Verification items for the finished model (mm, model axes). A direction names the side the tool comes from. Coordinates: 2 decimals unless noted, no trailing zeros. Order: outer loops, then holes, each group sorted by start corner. A loop starts at its lowest first (then second) coordinate and runs counter-clockwise, first axis right, second up. Notation, with made-up numbers: (9, 15.25) -> (45, 15.25) arc R25 ccw to (45, 29.25) -> close; hole circle Ø3 at (64.5, 34). An arc over 180 degrees is marked (long way). Use CSV: the item, a comma, the result in double quotes. Start each with the question number.
1) Scan lines: line 1 along X through (y, z) = (-4.5, 1.5); line 2 along Y through (x, z) = (10, 0.5); line 3 along X through (y, z) = (18, 1.75). Record each from-to range of solid material in increasing order.
2) Sectioned sample at A-A on x = 10. Record the boundary of the cut face in (y, z).
3) Go/stop test with flat-tipped pins: pin 1 (2.5 mm diameter, centred on x = -18.43, y = 21.91, fed in from +Z); pin 2 (1.8 mm diameter, centred on x = -18.43, y = -4.09, fed in from +Z); pin 3 (0.8 mm diameter, centred on x = -7.5, z = 0.5, fed in from -Y). Record where each tip stops, or that it passes through.
4) Tool access check on faces 1 (the flat face through (-1.103, -0.079, 0.986)), 2 (the cylindrical face through (14.774, -7.935, 1.699)), 3 (the cylindrical face through (17.6, -8.808, 1.699)). Record the directions out of +Z, -Z, +X, -X, +Y, -Y that give a thin tool (end or side, any length) a straight path to the whole face; none if there is none.
5) Sectioned sample at B-B on z = 1.7. Give the number of separate pieces and of enclosed holes in the cut face, then the cut area to 3 significant figures.
6) Release check for a two-part mould opening along X. For faces 4 (the cylindrical face through (-19.456, -8.808, 1.699)), 5 (the flat face through (-16.6, -8.3, 0.5)), 6 (the cylindrical face through (10.59, -3.31, 0.99)), 7 (the flat face through (19.572, 8.1, 0.5)) record: released by +X, released by -X, zero draft, split by the parting line, or undercut.
7) Sectioned sample at C-C on y = 0. Record the boundary of the cut face in (x, z), then the cut area to 3 significant figures.
from build123d import *

# Parameters (mm, degrees)
SKETCH_1_R          = 1.1
SKETCH_1_W          = 21
SKETCH_1_H          = 14
EXTRUDE_1_DEPTH     = 2
FILLET_2_R          = 1
SKETCH_11_R         = 1
CUT_EXTRUDE_1_DEPTH = 33.917032345
CHAMFER_1_SIZE      = 2


with BuildPart() as part:
    # 草图1 → 凸台-拉伸1 (new body)
    with BuildSketch(Plane.XY):
        Polygon((-21.428351104, 24.906962627), (19.571648896, 24.906962627), (19.571648896, -9.093037373), (17.69677195, -9.093037373), (15.571648896, -9.093037373), (13.89965532, -7.493037373), (-15.756357529, -7.493037373), (-17.428351104, -9.093037373), (-21.428351104, -9.093037373), align=None)
        with Locations((-11.428351104, 18.906962627)):
            Circle(SKETCH_1_R, mode=Mode.SUBTRACT)
        with Locations((-11.428351104, -2.893037373)):
            Circle(SKETCH_1_R, mode=Mode.SUBTRACT)
        with Locations((9.571648896, 18.906962627)):
            Circle(SKETCH_1_R, mode=Mode.SUBTRACT)
        with Locations((9.571648896, -2.893037373)):
            Circle(SKETCH_1_R, mode=Mode.SUBTRACT)
        with Locations((-0.928351104, 7.906962627)):
            Rectangle(SKETCH_1_W, SKETCH_1_H, mode=Mode.SUBTRACT)
    extrude(amount=EXTRUDE_1_DEPTH)

    # 圆角2
    fillet_2_edges = [part.edges().sort_by_distance(p)[0] for p in [
        (-16.592354317, -8.293037373, 2),
        (-0.928351104, -7.493037373, 2),
        (14.735652108, -8.293037373, 2),
        (17.571648896, -9.093037373, 2),
        (19.571648896, 7.906962627, 2),
        (-0.928351104, 24.906962627, 2),
        (-21.428351104, 7.906962627, 2),
        (-19.428351104, -9.093037373, 2),
    ]]
    fillet(fillet_2_edges, radius=FILLET_2_R)

    # 草图11 → 切除-拉伸1 (cut, through all)
    with BuildSketch(Plane.XY.offset(2)):
        with Locations((-18.428351104, 21.906962627)):
            Circle(SKETCH_11_R)
        with Locations((-18.428351104, -4.093037373)):
            Circle(SKETCH_11_R)
        with Locations((16.571648896, 21.906962627)):
            Circle(SKETCH_11_R)
        with Locations((16.571648896, -4.093037373)):
            Circle(SKETCH_11_R)
    extrude(amount=-CUT_EXTRUDE_1_DEPTH, mode=Mode.SUBTRACT)

    # 倒角1
    chamfer_1_edges = [part.edges().sort_by_distance(p)[0] for p in [
        (-0.928351104, 0.906962627, 2),
        (9.571648896, 7.906962627, 2),
        (-11.428351104, 7.906962627, 2),
        (-0.928351104, 14.906962627, 2),
    ]]
    chamfer(chamfer_1_edges, length=CHAMFER_1_SIZE - 0.0001)  # a hair under: the kernel refuses the full size


solid = part.part
Answers follow:
1,line 1,"x = -21.29 to -19.34, -17.51 to 15.66, 17.49 to 19.44"
1,line 2,"y = -7.49 to -3.91, -1.88 to 0.41, 15.41 to 17.89, 19.92 to 24.91"
1,line 3,"x = -21.09 to -12.05, -10.81 to 8.95, 10.19 to 19.23"
2,outline,"(-7.49, 0) -> (-3.91, 0) -> (-3.91, 2) -> (-6.49, 2) arc R1 ccw to (-7.49, 1) -> close; (-1.88, 0) -> (17.89, 0) -> (17.89, 2) -> (16.91, 2) -> (15.34, 0.43) -> (0.48, 0.43) -> (-1.09, 2) -> (-1.88, 2) -> close; (19.92, 0) -> (24.91, 0) -> (24.91, 1) arc R1 ccw to (23.91, 2) -> (19.92, 2) -> close"
3,pin 1,"stops at z = 2"
3,pin 2,"passes through"
3,pin 3,"stops at y = -7.49"
4,face 1,"+Z"
4,face 2,"+Z, -Y"
4,face 3,"+Z, +X, -X, -Y"
5,separate pieces,"1"
5,enclosed holes,"9"
5,area,"849 mm²"
6,face 4,"zero draft"
6,face 5,"undercut"
6,face 6,"undercut"
6,face 7,"released by +X"
7,outline,"(-21.43, 0) -> (19.57, 0) -> (19.57, 1) arc R1 ccw to (18.57, 2) -> (11.57, 2) -> (10.48, 0.91) -> (-12.34, 0.91) -> (-13.43, 2) -> (-20.43, 2) arc R1 ccw to (-21.43, 1) -> close"
7,area,"55.4 mm²"
